Could you check a few things on this drawing? It's one solid part, dimensions in mm from its lowest x, y, z. A direction names the side the tool comes from. Give positions to 0.01 mm unless a question says otherwise; leave off trailing zeros. Order: outer loops, then holes, each group sorted by start corner. A loop starts at its lowest first (then second) coordinate and runs counter-clockwise, first axis right, second up. Notation, with made-up numbers: (-35.75, 1) - (-3.75, 1) arc R25 ccw to (-3.75, 18) - close; hole circle Ø1 at (77.25, 85). An arc over 180 degrees is marked (long way). Return JSON: item names as keys, results as strings.
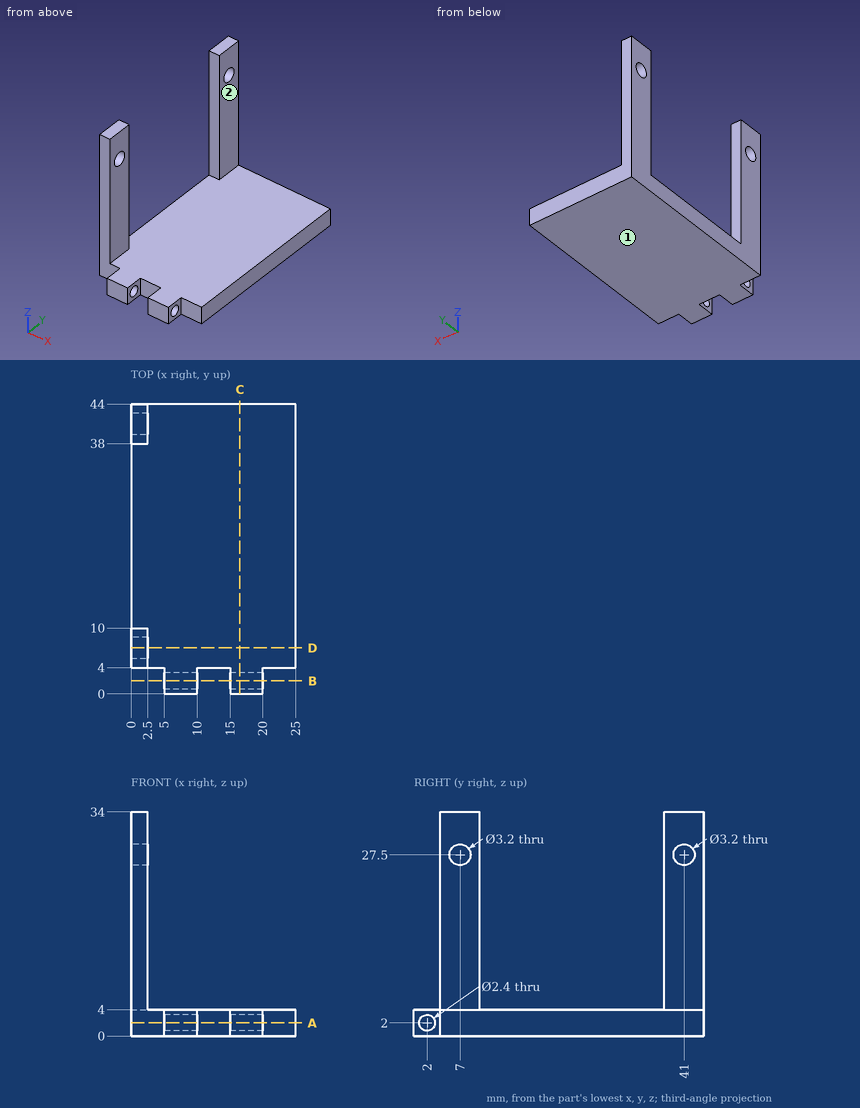
1. Suppose I cut it at B-B (y = 2). List the corners of the cut face in (x, z) for me, plus the area to 3 significant figures.
Checks:
{"outline": "(5, 0) - (10, 0) - (10, 0.8) - (5, 0.8) - close; (5, 3.2) - (10, 3.2) - (10, 4) - (5, 4) - close; (15, 0) - (20, 0) - (20, 0.8) - (15, 0.8) - close; (15, 3.2) - (20, 3.2) - (20, 4) - (15, 4) - close", "area": "16.0 mm^2"}
2. Suppose I cut it at A-A (z = 2). List the corners of the cut face in (x, y) for me, plus the area to 3 significant figures.
Checks:
{"outline": "(0, 4) - (5, 4) - (5, 3.2) - (10, 3.2) - (10, 4) - (15, 4) - (15, 3.2) - (20, 3.2) - (20, 4) - (25, 4) - (25, 44) - (0, 44) - close; (5, 0) - (10, 0) - (10, 0.8) - (5, 0.8) - close; (15, 0) - (20, 0) - (20, 0.8) - (15, 0.8) - close", "area": "1,020 mm^2"}
3. Suppose I cut it at C-C (x = 16.5). List the corners of the cut face in (y, z) for me, plus the area to 3 significant figures.
Checks:
{"outline": "(0, 0) - (44, 0) - (44, 4) - (0, 4) - close; hole circle Ø2.4 at (2, 2)", "area": "171 mm^2"}
4. On a 3-axis mill with a long thin cutter (end or side, diameter ignored), from which of +Z, -Z, +X, -X, +Y, -Y can I reach the whole of each face in a straight line? I mean the marked faces 1 and 2. Say none if no direction works.
Checks:
{"face 1": "-Z, +X, -X, +Y, -Y", "face 2": "+Z, +X, +Y, -Y"}
5. Suppose I cut it at D-D (y = 7). List the corners of the cut face in (x, z) for me.
Checks:
{"outline": "(0, 0) - (25, 0) - (25, 4) - (2.5, 4) - (2.5, 25.9) - (0, 25.9) - close; (0, 29.1) - (2.5, 29.1) - (2.5, 34) - (0, 34) - close"}
6. If I drill on L1, parallel to Z at x = 1.35, y = 7; L2, parallel to Z at x = 9.5, y = 41; L3, parallel to X at y = 7.5, z = 14, over which ranges is the centre line in solid material (lowest first)? Write a range as [from, to].
Checks:
{"L1": "[0, 25.9], [29.1, 34]", "L2": "[0, 4]", "L3": "[0, 2.5]"}
7. For pin 1 Ø4 at (y, z) = (7, 27.5) entering from +X; pin 2 Ø12 at (x, y) = (10, 31.5) entering from +Z; pin 3 Ø1.9 at (y, z) = (2, 2) entering from +X; pin 4 Ø1.5 at (x, z) = (2, 21) entering from -Y, each with a flat end and sliding along its axis, tell me the tip position at first contact or that it passes through.
Checks:
{"pin 1": "x = 2.5", "pin 2": "z = 4", "pin 3": "through", "pin 4": "y = 4"}
